```python
from build123d import *

# Parameters (mm, degrees)
SKETCH_1_R               = 59
SKETCH_1_R_2             = 11.1
EXTRUDE_1_DEPTH          = 6
SKETCH_2_R               = 1.525
CUT_EXTRUDE_1_DEPTH      = 6
EXTRUDE_START            = -6
EXTRUDE_2_DEPTH          = 6
SKETCH_4_R               = 4.2
SKETCH_4_R_2             = 2.025
CUT_EXTRUDE_2_DEPTH      = 6
SKETCH_5_R               = 4.2
CUT_EXTRUDE_3_DEPTH      = 6
CUT_EXTRUDE_4_DEPTH      = 10
CUT_EXTRUDE_5_DEPTH      = 10
CUT_EXTRUDE_7_DEPTH      = 10
FILLET_1_R               = 3
SKETCH_11_R              = 2.5
CUT_EXTRUDE_8_DEPTH      = 10
CUT_EXTRUDE_9_DEPTH      = 10
PATTERN_CIRCULAR_1_COUNT = 3
CUT_EXTRUDE_10_DEPTH     = 20
FILLET_3_R               = 20
FILLET_4_R               = 2


with BuildPart() as part:
    # 草图1 → 凸台-拉伸1 (new body)
    with BuildSketch(Plane(origin=(0, 0, 0), x_dir=(1, 0, 0), z_dir=(0, 1, 0))):
        with Locations(Location((0, 0, 0), (0, 0, 270))):
            Circle(SKETCH_1_R)
        with Locations(Location((0, 0, 0), (0, 0, 270))):
            Circle(SKETCH_1_R_2, mode=Mode.SUBTRACT)
    extrude(amount=EXTRUDE_1_DEPTH)

    # 草图2 → 切除-拉伸1 (cut)
    with BuildSketch(Plane(origin=(0, 6, 0), x_dir=(1, 0, 0), z_dir=(0, 1, 0))):
        with Locations(Location((0, 56, 0), (0, 0, 270))):
            Circle(SKETCH_2_R)
        with Locations(Location((39.597979746, 39.597979746, 0), (0, 0, 270))):
            Circle(SKETCH_2_R)
        with Locations(Location((56, 0, 0), (0, 0, 270))):
            Circle(SKETCH_2_R)
        with Locations(Location((39.597979746, -39.597979746, 0), (0, 0, 270))):
            Circle(SKETCH_2_R)
        with Locations(Location((0, -56, 0), (0, 0, 270))):
            Circle(SKETCH_2_R)
        with Locations(Location((-39.597979746, -39.597979746, 0), (0, 0, 270))):
            Circle(SKETCH_2_R)
        with Locations(Location((-56, 0, 0), (0, 0, 270))):
            Circle(SKETCH_2_R)
        with Locations(Location((-39.597979746, 39.597979746, 0), (0, 0, 270))):
            Circle(SKETCH_2_R)
    extrude(amount=-CUT_EXTRUDE_1_DEPTH, mode=Mode.SUBTRACT)

    # 草图3 → 凸台-拉伸2 (add)
    with BuildSketch(Plane(origin=(0, 6, 0), x_dir=(1, 0, 0), z_dir=(0, 1, 0)).offset(EXTRUDE_START)):
        with BuildLine():
            Line((-51.088050573, 29.512896989), (-22.5, 79))
            Line((-22.5, 79), (22.5, 79))
            Line((22.5, 79), (51.088050573, 29.512896989))
            ThreePointArc((51.088050573, 29.512896989), (0, 59), (-51.088050573, 29.512896989))
        make_face()
    extrude(amount=EXTRUDE_2_DEPTH)

    # 草图4 → 切除-拉伸2 (cut)
    with BuildSketch(Plane.XZ):
        with Locations(Location((0, 19.25, 0), (0, 0, 270))):
            Circle(SKETCH_4_R)
        with Locations(Location((0, 29, 0), (0, 0, 270))):
            Circle(SKETCH_4_R_2)
        with Locations(Location((25.11473671, -14.5, 0), (0, 0, 270))):
            Circle(SKETCH_4_R_2)
        with Locations(Location((-25.11473671, -14.5, 0), (0, 0, 270))):
            Circle(SKETCH_4_R_2)
    extrude(amount=-CUT_EXTRUDE_2_DEPTH, mode=Mode.SUBTRACT)

    # 草图5 → 切除-拉伸3 (cut)
    with BuildSketch(Plane.XZ):
        with Locations(Location((16.02146997, 9.25, 0), (0, 0, 270))):
            Circle(SKETCH_5_R)
    extrude(amount=-CUT_EXTRUDE_3_DEPTH, mode=Mode.SUBTRACT)

    # 草图8 → 切除-拉伸4 (cut)
    with BuildSketch(Plane.XZ):
        with BuildLine():
            Line((38.990090266, -27.129741264), (26.368115905, -19.842440969))
            ThreePointArc((26.368115905, -19.842440969), (0, -33), (-26.368115905, -19.842440969))
            Line((-26.368115905, -19.842440969), (-38.990090266, -27.129741264))
            ThreePointArc((-38.990090266, -27.129741264), (0, -47.5), (38.990090266, -27.129741264))
        make_face()
    extrude(amount=-CUT_EXTRUDE_4_DEPTH, mode=Mode.SUBTRACT)

    # 草图9 → 切除-拉伸5 (cut)
    with BuildSketch(Plane.XZ):
        with BuildLine():
            ThreePointArc((34, 0), (33.302950494, -6.849342188), (31.240383034, -13.417841401))
            Line((31.240383034, -13.417841401), (42.990090266, -20.201538034))
            ThreePointArc((42.990090266, -20.201538034), (46.35881409, -10.349413326), (47.5, 0))
            ThreePointArc((47.5, 0), (34.973204028, 32.142261899), (4, 47.331279298))
            Line((4, 47.331279298), (4, 33.763886032))
            ThreePointArc((4, 33.763886032), (25.416530054, 22.583179581), (34, 0))
        make_face()
    extrude(amount=-CUT_EXTRUDE_5_DEPTH, mode=Mode.SUBTRACT)

    # 草图10 → 切除-拉伸7 (cut)
    with BuildSketch(Plane.XZ):
        with BuildLine():
            Line((-42.990090266, -20.201538034), (-31.240383034, -13.417841401))
            ThreePointArc((-31.240383034, -13.417841401), (-30.175452448, 15.666590872), (-7, 33.271609519))
            Line((-7, 33.271609519), (-7, 46.98137929))
            ThreePointArc((-7, 46.98137929), (-41.870495295, 22.430149883), (-42.990090266, -20.201538034))
        make_face()
    extrude(amount=-CUT_EXTRUDE_7_DEPTH, mode=Mode.SUBTRACT)

    # 圆角1
    fillet_1_edges = [part.edges().sort_by_distance(p)[0] for p in [
        (42.990090266, 3, -20.201538034),
        (31.240383034, 3, -13.417841401),
        (4, 3, 33.763886032),
        (4, 3, 47.331279298),
        (-7, 3, 46.98137929),
        (-7, 3, 33.271609519),
        (-31.240383034, 3, -13.417841401),
        (-42.990090266, 3, -20.201538034),
        (-26.368115905, 3, -19.842440969),
        (26.368115905, 3, -19.842440969),
        (38.990090266, 3, -27.129741264),
        (-38.990090266, 3, -27.129741264),
    ]]
    fillet(fillet_1_edges, radius=FILLET_1_R)

    # 草图11 → 切除-拉伸8 (cut)
    with BuildSketch(Plane(origin=(0, 6, 0), x_dir=(1, 0, 0), z_dir=(0, 1, 0))):
        with Locations(Location((15, 63, 0), (0, 0, 270))):
            Circle(SKETCH_11_R)
        with Locations(Location((15, 74, 0), (0, 0, 270))):
            Circle(SKETCH_11_R)
        with Locations(Location((-15, 63, 0), (0, 0, 270))):
            Circle(SKETCH_11_R)
        with Locations(Location((-15, 74, 0), (0, 0, 270))):
            Circle(SKETCH_11_R)
    extrude(amount=-CUT_EXTRUDE_8_DEPTH, mode=Mode.SUBTRACT)

    # 草图12 → 切除-拉伸9 (cut)
    with BuildSketch(Plane.XZ):
        with BuildLine():
            ThreePointArc((-11.126662137, -24.600759941), (3.851051224, -26.723948145), (17.619884076, -20.458242475))
            ThreePointArc((17.619884076, -20.458242475), (18.140249782, -13.477252607), (11.159259915, -12.956886901))
            ThreePointArc((11.159259915, -12.956886901), (2.438999108, -16.925167159), (-7.04688602, -15.580481296))
            ThreePointArc((-7.04688602, -15.580481296), (-13.596913401, -18.05073256), (-11.126662137, -24.600759941))
        make_face()
    cut_extrude_9 = extrude(amount=-CUT_EXTRUDE_9_DEPTH, mode=Mode.SUBTRACT)

    # 阵列(圆周)1: 切除-拉伸9 ×3 about axis, 1 skipped
    pattern_circular_1_axis = Axis((0, 0, 0), (0, 1, 0))
    add([cut_extrude_9.rotate(pattern_circular_1_axis, i * 360 / PATTERN_CIRCULAR_1_COUNT) for i in range(1, PATTERN_CIRCULAR_1_COUNT) if i not in (2,)], mode=Mode.SUBTRACT)

    # 草图15 → 切除-拉伸10 (cut, symmetric)
    with BuildSketch(Plane.XZ):
        with BuildLine():
            Line((22.5, -79), (22.5, -69))
            Line((22.5, -69), (47.535137175, -34.948687153))
            ThreePointArc((47.535137175, -34.948687153), (49.386437856, -32.279711212), (51.088050573, -29.512896989))
            Line((51.088050573, -29.512896989), (22.5, -79))
        make_face()
        with BuildLine():
            Line((-22.5, -79), (-51.088050573, -29.512896989))
            ThreePointArc((-51.088050573, -29.512896989), (-49.386437856, -32.279711212), (-47.535137175, -34.948687153))
            Line((-47.535137175, -34.948687153), (-22.5, -69))
            Line((-22.5, -69), (-22.5, -79))
        make_face()
    extrude(amount=CUT_EXTRUDE_10_DEPTH, both=True, mode=Mode.SUBTRACT)

    # 圆角3
    fillet_3_edges = [part.edges().sort_by_distance(p)[0] for p in [
        (-22.5, 3, -69),
        (22.5, 3, -69),
    ]]
    fillet(fillet_3_edges, radius=FILLET_3_R)

    # 圆角4
    fillet_4_edges = [part.edges().sort_by_distance(p)[0] for p in [
        (-22.5, 3, -79),
        (22.5, 3, -79),
    ]]
    fillet(fillet_4_edges, radius=FILLET_4_R)


solid = part.part
```
Geometry check sheet. Reference: the model listing, model coordinates, mm. Give positions to 0.01 mm unless a question says otherwise; leave off trailing zeros. Order: outer loops, then holes, each group sorted by start corner. A loop starts at its lowest first (then second) coordinate and runs counter-clockwise, first axis right, second up. Notation, with made-up numbers: (-8, 50.5) - (47, 50.5) arc R18 cw to (47, 74.5) - close; hole circle Ø8 at (2.25, 68). An arc over 180 degrees is marked (long way). Write item = value, one per line. Start each with the question number.
1) Section check A-A (x = 0). Count the separate pieces of the cut face and the enclosed holes in it, then the cut area to 3 significant figures.
2) Draft check along Z on faces 1 (the flat face through (-37.11, 2.96, -49.13)), 2 (the cylindrical face through (14.04, 3.04, -60.69)). Enter one of: released by +Z, released by -Z, zero draft, split by the parting line, or undercut.
3) Section check C-C (z = -56). Enter the section's corners in (x, y) (3 decimals), then the cut area to 3 significant figures.
4) Gauge pin test, flat ends, axial feed: pin 1 Ø9.5 at (x, z) = (0, 19.25) entering from +Y; pin 2 Ø2 at (y, z) = (1, 29) entering from -X; pin 3 Ø0.7 at (y, z) = (3, -76.5) entering from -X; pin 4 Ø1.8 at (y, z) = (2.5, 39.5) entering from -X. Record the tip position at first contact, or that the pin passes through.
5) Section check D-D (x = 56). Enter the section's corners in (y, z) (3 decimals), then the cut area to 3 significant figures.
6) Scan lines: L1, parallel to Z at x = 28, y = 3.25; L2, parallel to Z at x = 10, y = 3.25; L3, parallel to X at y = 5.5, z = 26. Record each from-to range of solid material in increasing order.
7) Section check B-B (z = -74). Enter the section's corners in (x, y).
Geometry check:
q1.separate_pieces = 8
q1.enclosed_holes = 0
q1.area = 437 mm2
q2.face_1 = released by -Z
q2.face_2 = undercut
q3.outline = (-32.058, 0) - (-1.525, 0) - (-1.525, 6) - (-32.058, 6) - close; (1.525, 0) - (32.058, 0) - (32.058, 6) - (1.525, 6) - close
q3.area = 366 mm2
q4.pin_1 = 6
q4.pin_2 = -51.93
q4.pin_3 = -22.5
q4.pin_4 = -44.62
q5.outline = (0, -18.574) - (6, -18.574) - (6, -1.525) - (0, -1.525) - close; (0, 1.525) - (6, 1.525) - (6, 18.574) - (0, 18.574) - close
q5.area = 205 mm2
q6.L1 = -61.52 to -38.37, -20.86 to 19.29, 38.37 to 51.93
q6.L2 = -79 to -46.44, -31.45 to -25.08, -13.87 to -4.82, 4.82 to 32.5, 46.44 to 58.15
q6.L3 = -52.96 to -39.75, -21.91 to 21.91, 39.75 to 52.96
q7.outline = (-22.56, 0) - (-17.5, 0) - (-17.5, 6) - (-22.56, 6) - close; (-12.5, 0) - (12.5, 0) - (12.5, 6) - (-12.5, 6) - close; (17.5, 0) - (22.56, 0) - (22.56, 6) - (17.5, 6) - close
